Answer from the drawing. Dimensions are ordinates in mm from the lowest x, y and z of the part. A direction names the side the tool comes from. Coordinates: 2 decimals unless noted, no trailing zeros. Order: outer loops, then holes, each group sorted by start corner. A loop starts at its lowest first (then second) coordinate and runs counter-clockwise, first axis right, second up. Notation, with made-up numbers: (23, 46.25) -> (79, 46.25) arc R27 cw to (79, 69.25) -> close; hole circle Ø4 at (11.25, 5). An arc over 180 degrees is marked (long way). Use CSV: the item, a comma, the result in double quotes.
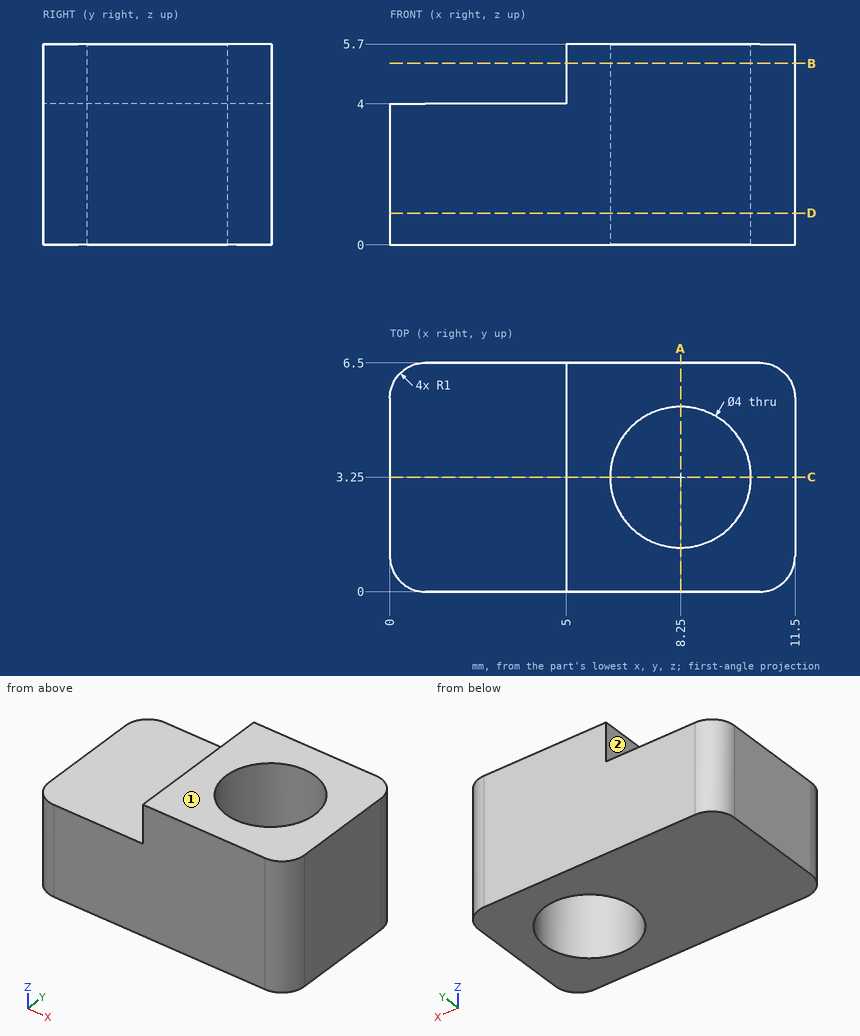
Item 1: Each of these flat-tipped pins is pushed along its axis until it touches: P1, Ø2.5, axis at x = 1.5, y = 3.5, coming from the +Z side; P2, Ø1.5, axis at x = 8.5, y = 5, coming from the -Z side; P3, Ø0.8, axis at y = 4, z = 4.5, coming from the -X side. Where does it stop, or does it pass through?
Return value:
P1,"stops at z = 4"
P2,"stops at z = 0"
P3,"stops at x = 5"
Item 2: Find section A-A, the plane x = 8.25. Give the vertices of the cut face in (y, z).
Return value:
outline,"(0, 0) -> (1.25, 0) -> (1.25, 5.7) -> (0, 5.7) -> close; (5.25, 0) -> (6.5, 0) -> (6.5, 5.7) -> (5.25, 5.7) -> close"
Item 3: A tool of negligible diameter and unlimited length cuts with its end or side. For the marked faces 1 and 2, from which of +Z, -Z, +X, -X, +Y, -Y can it reach the whole face along a straight path? Write none if from no direction.
Return value:
face 1,"+Z, +X, -X, +Y, -Y"
face 2,"+Z, -X, +Y, -Y"
Item 4: Find section C-C, the plane y = 3.25. Give the vertices of the cut face in (x, z), then the cut area to 4 significant figures.
Return value:
outline,"(0, 0) -> (6.25, 0) -> (6.25, 5.7) -> (5, 5.7) -> (5, 4) -> (0, 4) -> close; (10.25, 0) -> (11.5, 0) -> (11.5, 5.7) -> (10.25, 5.7) -> close"
area,"34.25 mm^2"
Item 5: Find section D-D, the plane z = 0.9. Give the vertices of the cut face in (x, y), then the cut area to 3 significant figures.
Return value:
outline,"(0, 1) arc R1 ccw to (1, 0) -> (10.5, 0) arc R1 ccw to (11.5, 1) -> (11.5, 5.5) arc R1 ccw to (10.5, 6.5) -> (1, 6.5) arc R1 ccw to (0, 5.5) -> close; hole circle Ø4 at (8.25, 3.25)"
area,"61.3 mm^2"
Item 6: Find section B-B, the plane z = 5.15. Give the vertices of the cut face in (x, y).
Return value:
outline,"(5, 0) -> (10.5, 0) arc R1 ccw to (11.5, 1) -> (11.5, 5.5) arc R1 ccw to (10.5, 6.5) -> (5, 6.5) -> close; hole circle Ø4 at (8.25, 3.25)"
Item 7: Straight lines are drawn through the part: line 1 along Y through (x, z) = (8.25, 5); line 2 along X through (y, z) = (3.25, 4.5); line 3 along X through (y, z) = (3.25, 1.7). For each, find the intervals that lie inside material, in ascending order.
Return value:
line 1,"y = 0 to 1.25, 5.25 to 6.5"
line 2,"x = 5 to 6.25, 10.25 to 11.5"
line 3,"x = 0 to 6.25, 10.25 to 11.5"
